Autodesk Inventor part; units mm, degrees
ref_plane "YZ Plane" through (0, 0, 0) normal (1, 0, 0) x (0, 1, 0)
ref_plane "XZ Plane" through (0, 0, 0) normal (0, 1, 0) x (-1, 0, 0)
ref_plane "XY Plane" through (0, 0, 0) normal (0, 0, 1) x (1, 0, 0)
sketch "Sketch1" plane through (0, 0, 0) normal (0, 1, 0) x (-1, 0, 0)
  line L0 (0, 0) -> (40, 0)
  line L1 (40, 0) -> (40, -3)
  line L2 (40, -3) -> (0, -3)
  line L3 (0, -3) -> (0, 0)
  line L4 (0, 0) -> (3, 0)
  line L5 (3, 0) -> (3, -34)
  line L6 (3, -34) -> (0, -34)
  line L7 (0, -34) -> (0, 0)
  dimension "d0" = 3
  dimension "d1" = 3
  dimension "d2" = 40
  dimension "d3" = 34
extrude "Extrusion1" add sketch "Sketch1" along normal blind 15
fillet "Fillet1" radius 2 1 edges at (-3, 7.5, -3)
fillet "Fillet2" radius 5 1 edges at (0, 7.5, 0)
sketch "Sketch3" plane through (-40, 0, -3) normal (0, 0, -1) x (-1, 0, 0)
  line L0 (-35, 15) -> (0, 15)
  line L1 (-35, 0) -> (0, 0)
  line L2 (0, 0) -> (0, 15)
  line L3 (-40, 0) -> (-40, 15)
  line L4 (-40, 0) -> (-40, 15)
  point P0 (-7.5, 7.5)
  point P1 (-27.5, 7.5)
  dimension "d20" = 7.5
  dimension "d29" = 7.5
  dimension "d33" = 12.5
hole "Hole2" at (-32.5, 7.5, -3) at (-12.5, 7.5, -3) direction (0, 0, 1) diameter 4.5 end through all
equation "\"d1\" = d0"
properties part number "Pancake_Floor Bracket" material "Aluminum 6061"
Input: part model. Units: mm. Frame: model coordinates. A direction names the side the tool comes from. Coordinates: 2 decimals unless noted, no trailing zeros. Loops run counter-clockwise (first coordinate to the right, second up) from the corner with the lowest first, then second, coordinate; pieces in that order, holes last.
(1) Section B-B on x = -12.5. Return the cut outline in (y, z), then the cut area to 3 significant figures.
(2) First-contact query: pin 1 Ø2.5 at (x, y) = (-12.5, 7.5) entering from +Z; pin 2 Ø1 at (x, y) = (-26, 9) entering from -Z; pin 3 Ø6 at (y, z) = (4.5, -12) entering from -X. Flat tips, straight axial feed; report the tip coordinate or a pass-through.
(3) Section C-C on z = -19. Return the cut outline in (x, y).
(4) Section A-A on y = 7.5. Return the cut outline in (x, z).
(5) Material intervals for probe 1 along Y at (x, z) = (-32.5, -0.7); probe 2 along X at (y, z) = (7.5, -0.8); probe 3 along X at (y, z) = (7.5, -1.9), sorted ascending.
(6) Section D-D on x = -8.5. Return the cut outline in (y, z).
(7) Pull-direction query (Y, two-part tool) for faces 3 (the face through (-14.73, 7.21, -1.48)), 4 (the face through (-34.73, 7.21, -1.48)), 5 (the face through (-11, 0, -2)), 6 (the face through (-40, 7, -1)); classes: released by +Y, released by -Y, zero draft, split by the parting line, or undercut.
(8) Set-up query: faces 1 (the face through (-3, 7, -19)), 2 (the face through (-2, 8, -1)). Return all of +Z, -Z, +X, -X, +Y, -Y with unobstructed straight access to the full face (end or side cutting, diameter ignored); none if empty.
Data:
1. outline: (0, -3) - (5.25, -3) - (5.25, 0) - (0, 0) - close; (9.75, -3) - (15, -3) - (15, 0) - (9.75, 0) - close
1. area: 31.5 mm2
2. pin 1: passes through
2. pin 2: stops at z = -3
2. pin 3: stops at x = -3
3. outline: (-3, 0) - (0, 0) - (0, 15) - (-3, 15) - close
4. outline: (-40, -3) - (-34.75, -3) - (-34.75, 0) - (-40, 0) - close; (-30.25, -3) - (-14.75, -3) - (-14.75, 0) - (-30.25, 0) - close; (-10.25, -3) - (-5, -3) arc R2 cw to (-3, -5) - (-3, -34) - (0, -34) - (0, -5) arc R5 ccw to (-5, 0) - (-10.25, 0) - close
5. probe 1: y = 0 to 5.25, 9.75 to 15
5. probe 2: x = -40 to -34.75, -30.25 to -14.75, -10.25 to -2.29
5. probe 3: x = -40 to -34.75, -30.25 to -14.75, -10.25 to -1.08
6. outline: (0, -3) - (15, -3) - (15, 0) - (0, 0) - close
7. face 3: undercut
7. face 4: undercut
7. face 5: released by -Y
7. face 6: zero draft
8. face 1: -Z, -X, +Y, -Y
8. face 2: +Z, +X, +Y, -Y
